CAD build for the part. Positions are in the model's coordinates, mm. Face numbers are marked on the shaded views. A direction names the side the tool comes from. Round coordinates to 2 decimals unless told otherwise and drop trailing zeros. Loops run counter-clockwise (first coordinate to the right, second up) from the corner with the lowest first, then second, coordinate; pieces in that order, holes last.
Autodesk Inventor part; units mm, degrees
ref_plane "YZ Plane" through (0, 0, 0) normal (1, 0, 0) x (0, 1, 0)
ref_plane "XZ Plane" through (0, 0, 0) normal (0, 1, 0) x (-1, 0, 0)
ref_plane "XY Plane" through (0, 0, 0) normal (0, 0, 1) x (1, 0, 0)
sketch "Sketch1" plane through (0, 0, 0) normal (0, 0, 1) x (1, 0, 0)
  line L0 (24.7, 16.2) -> (24.7, -16.2)
  line L1 (24.7, -16.2) -> (-24.7, -16.2)
  line L2 (-24.7, -16.2) -> (-24.7, 16.2)
  line L3 (-24.7, 16.2) -> (24.7, 16.2)
  arc A0 (26.5, 15) -> (23.5, 18) centre (23.5, 15) ccw
  line L4 (23.5, 18) -> (-23.5, 18)
  arc A1 (-23.5, 18) -> (-26.5, 15) centre (-23.5, 15) ccw
  line L5 (-26.5, 15) -> (-26.5, -15)
  arc A2 (-26.5, -15) -> (-23.5, -18) centre (-23.5, -15) ccw
  line L6 (-23.5, -18) -> (23.5, -18)
  arc A3 (23.5, -18) -> (26.5, -15) centre (23.5, -15) ccw
  line L7 (26.5, -15) -> (26.5, 15)
  point P0 (0, 0)
extrude "Extrusion1" add sketch "Sketch1" along normal blind 1.8 contours L0 L1 L2 L3 | L7 A3 L6 A2 L5 A1 L4 A0
sketch "Sketch2" plane through (0, 0, 1.8) normal (0, 0, 1) x (1, 0, 0)
  circle A0 centre (-18.5, 0) radius 1.3
  circle A1 centre (18.5, 0) radius 1.3
  point P0 (0, 0)
extrude "Extrusion2" cut sketch "Sketch2" against normal blind 1.8
sketch "Sketch3" plane through (0, 0, 0) normal (0, 0, -1) x (-1, 0, 0)
  circle A0 centre (18.5, 0) radius 1.3
  circle A1 centre (-18.5, 0) radius 1.3
  circle A2 centre (-18.5, 0) radius 3.5
  circle A3 centre (18.5, 0) radius 3.5
  point P0 (0, 0)
  dimension "d4" = 7
  dimension "d5" = 7
extrude "Extrusion3" add sketch "Sketch3" along normal blind 6.05
fillet "Fillet1" radius 1.8 8 edges at (-25.6213, 17.1213, 1.8) (-26.5, 0, 1.8) (-25.6213, -17.1213, 1.8) (0, -18, 1.8) (25.6213, -17.1213, 1.8) (26.5, 0, 1.8) (25.6213, 17.1213, 1.8) (0, 18, 1.8)
chamfer "Chamfer1" distance 2 angle 45 2 edges at (17.2, 0, 1.8) (-19.8, 0, 1.8)
properties part number "top"
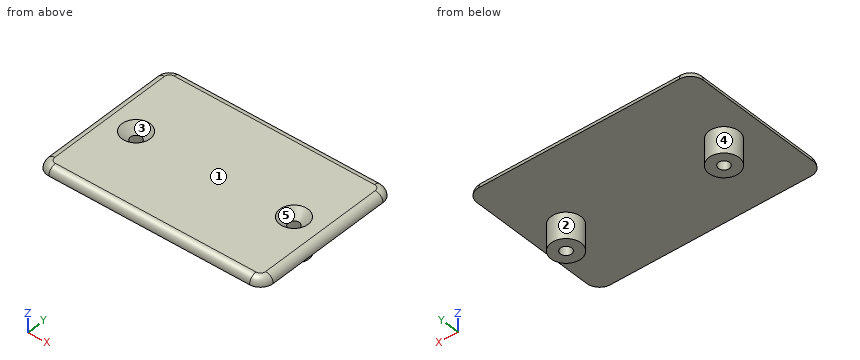
Item 1: Probe line 1 (Y direction, x = -18.5, z = -2.8); line 2 (Z direction, x = 8, y = -13.5); line 3 (X direction, y = 1, z = -5.25). List the from-to ranges inside material, lowest first.
Answers follow:
line 1: y = -3.5 to -1.3, 1.3 to 3.5
line 2: z = 0 to 1.8
line 3: x = -21.85 to -19.33, -17.67 to -15.15, 15.15 to 17.67, 19.33 to 21.85
Item 2: 3-axis set-ups, long thin cutter, end or side, ignore diameter. For the marked faces 4 and 5: which of +Z, -Z, +X, -X, +Y, -Y reach the whole face in a straight line?
Answers follow:
face 4: -Z
face 5: +Z
Item 3: Cut at B-B, the plane y = 0. State how many separate pieces and enclosed holes the cut face has, plus the area to 3 significant figures.
Answers follow:
separate pieces: 3
enclosed holes: 0
area: 130 mm2
Item 4: Two-plate mould, pull along X, no slides. Class the marked faces 1, 2 and 3: released by +X, released by -X, zero draft, split by the parting line, or undercut.
Answers follow:
face 1: zero draft
face 2: undercut
face 3: undercut
Item 5: Flat gauge pins, fed straight in: P1, Ø4, axis at y = -2.5, z = -0.5, coming from the +X side; P2, Ø8, axis at x = 2.5, y = 4, coming from the -Z side. Where does each tip first touch, or does it go through?
Answers follow:
P1: stops at x = 26.5
P2: stops at z = 0
Item 6: Cut at C-C, the plane z = -4. Give the cut face in (x, y).
Answers follow:
outline: circle Ø7 at (-18.5, 0); circle Ø7 at (18.5, 0); hole circle Ø2.6 at (-18.5, 0); hole circle Ø2.6 at (18.5, 0)
